from build123d import *

# Parameters (mm, degrees)
SKETCH1_W           = 584.2
SKETCH1_H           = 50.8
BOSS_EXTRUDE1_DEPTH = 9.525
SKETCH2_R           = 3.2639
CUT_EXTRUDE2_DEPTH  = 1390.972066491
SKETCH3_R           = 5.23875
CUT_EXTRUDE3_DEPTH  = 6.35
FILLET1_R           = 6.35
SKETCH4_R           = 2.4892
CUT_EXTRUDE4_DEPTH  = 1390.972066491
CHAMFER1_SIZE       = 0.79375
SHELL1_START        = 6.35
SHELL1_OUTLINE_R    = 8.8392
SHELL1_DEPTH        = 3.175


# Read off the part's stored shape, not the designer's step: Shell1
with BuildPart() as part:
    # Sketch1 → Boss-Extrude1 (new body)
    with BuildSketch(Plane.XY):
        with Locations((0, 1333.5)):
            Rectangle(SKETCH1_W, SKETCH1_H)
    extrude(amount=BOSS_EXTRUDE1_DEPTH)

    # Sketch2 → Cut-Extrude2 (cut, through all)
    with BuildSketch(Plane.XY):
        with Locations(Location((279.4, 1314.45, 0), (0, 0, 180))):
            Circle(SKETCH2_R)
        with Locations(Location((279.4, 1352.55, 0), (0, 0, 180))):
            Circle(SKETCH2_R)
    cut_extrude2 = extrude(amount=CUT_EXTRUDE2_DEPTH, mode=Mode.SUBTRACT)

    # Sketch3 → Cut-Extrude3 (cut)
    with BuildSketch(Plane(origin=(0, 0, 0), x_dir=(-1, 0, 0), z_dir=(0, 0, -1))):
        with Locations((-279.4, 1314.45)):
            Circle(SKETCH3_R)
        with Locations((-279.4, 1352.55)):
            Circle(SKETCH3_R)
    cut_extrude3 = extrude(amount=-CUT_EXTRUDE3_DEPTH, mode=Mode.SUBTRACT)

    # Fillet1
    fillet1_edges = [part.edges().sort_by_distance(p)[0] for p in [
        (292.1, 1308.1, 4.7625),
        (-292.1, 1308.1, 4.7625),
        (-292.1, 1358.9, 4.7625),
        (292.1, 1358.9, 4.7625),
    ]]
    fillet(fillet1_edges, radius=FILLET1_R)

    # Sketch4 → Cut-Extrude4 (cut, symmetric)
    with BuildSketch(Plane.XY):
        with Locations((150.8125, 1333.5)):
            Circle(SKETCH4_R)
        with Locations((188.9125, 1333.5)):
            Circle(SKETCH4_R)
    cut_extrude4 = extrude(amount=CUT_EXTRUDE4_DEPTH, both=True, mode=Mode.SUBTRACT)

    # Mirror2: Cut-Extrude2, Cut-Extrude3, Cut-Extrude4 across plane
    add(cut_extrude2.mirror(Plane(origin=(0, 0, 0), x_dir=(0, 0, 1), z_dir=(1, 0, 0))), mode=Mode.SUBTRACT)
    add(cut_extrude3.mirror(Plane(origin=(0, 0, 0), x_dir=(0, 0, 1), z_dir=(1, 0, 0))), mode=Mode.SUBTRACT)
    add(cut_extrude4.mirror(Plane(origin=(0, 0, 0), x_dir=(0, 0, 1), z_dir=(1, 0, 0))), mode=Mode.SUBTRACT)

    # Chamfer1
    chamfer1_edges = [part.edges().sort_by_distance(p)[0] for p in [
        (0, 1308.1, 0),
        (292.1, 1333.5, 0),
        (-292.1, 1333.5, 0),
        (0, 1358.9, 0),
        (290.240128061, 1357.040128061, 0),
        (290.240128061, 1309.959871939, 0),
        (-290.240128061, 1357.040128061, 0),
        (-290.240128061, 1309.959871939, 0),
    ]]
    chamfer(chamfer1_edges, length=CHAMFER1_SIZE)

    # Shell1 outline → Shell1 (cut)
    with BuildSketch(Plane.XY.offset(SHELL1_START)):
        with BuildLine():
            Line((285.75, 1324.144154247), (285.75, 1342.855845753))
            ThreePointArc((285.75, 1342.855845753), (273.89043722, 1342.354714593), (267.81125, 1352.55))
            Line((267.81125, 1352.55), (-267.81125, 1352.55))
            ThreePointArc((-267.81125, 1352.55), (-273.89043722, 1342.354714593), (-285.75, 1342.855845753))
            Line((-285.75, 1342.855845753), (-285.75, 1324.144154247))
            ThreePointArc((-285.75, 1324.144154247), (-273.89043722, 1324.645285407), (-267.81125, 1314.45))
            Line((-267.81125, 1314.45), (267.81125, 1314.45))
            ThreePointArc((267.81125, 1314.45), (273.89043722, 1324.645285407), (285.75, 1324.144154247))
        make_face()
        with Locations((-188.9125, 1333.5)):
            Circle(SHELL1_OUTLINE_R, mode=Mode.SUBTRACT)
        with Locations((-150.8125, 1333.5)):
            Circle(SHELL1_OUTLINE_R, mode=Mode.SUBTRACT)
        with Locations((150.8125, 1333.5)):
            Circle(SHELL1_OUTLINE_R, mode=Mode.SUBTRACT)
        with Locations((188.9125, 1333.5)):
            Circle(SHELL1_OUTLINE_R, mode=Mode.SUBTRACT)
    extrude(amount=SHELL1_DEPTH, mode=Mode.SUBTRACT)


solid = part.part
Check sheet for the modelled part. Datum: model origin and axes. Units: mm. A direction names the side the tool comes from. Round coordinates to 2 decimals unless told otherwise and drop trailing zeros. Order: outer loops, then holes, each group sorted by start corner. A loop starts at its lowest first (then second) coordinate and runs counter-clockwise, first axis right, second up.
Q1. Depth check by flat-ended pin: P1, Ø5, axis at x = -59.5, y = 1334.5, coming from the +Z side; P2, Ø4, axis at x = -279.4, y = 1352.55, coming from the -Z side; P3, Ø5, axis at x = 277.5, y = 1316, coming from the -Z side. Enter the tip coordinate at first touch or a pass-through.
Filled sheet:
P1: stops at z = 6.35
P2: passes through
P3: stops at z = 6.35
Q2. Set-up check for faces 1 (the face through (-277, 1355, 6.35)), 2 (the face through (-153, 1332, 9.525)), 3 (the face through (144.298, 1339.474, 7.915)): record each of +Z, -Z, +X, -X, +Y, -Y from which the full face is reachable in a straight line by a thin tool's end or side.
Filled sheet:
face 1: -Z
face 2: +Z, +X, -X, +Y, -Y
face 3: +Z
Q3. Draft check along Y on faces 4 (the face through (277, 1355, 6.35)), 5 (the face through (-1, 1313, 9.525)). Enter one of: pulls with the +Y half, pulls with the -Y half, needs draft (parallel to the pull), parting line crosses it, or undercut.
Filled sheet:
face 4: undercut
face 5: needs draft
Q4. Cross-section at B-B, the plane z = 3.75. Give the number of separate pieces and of enclosed holes in the cut face, plus the area to 3 significant figures.
Filled sheet:
separate pieces: 1
enclosed holes: 8
area: 29,200 mm2
Q5. Cross-section at A-A, the plane x = 67. Enter the section's corners in (y, z) (3 decimals), plus the area to 3 significant figures.
Filled sheet:
outline: (1308.1, 0.794) - (1308.894, 0) - (1358.106, 0) - (1358.9, 0.794) - (1358.9, 9.525) - (1352.55, 9.525) - (1352.55, 6.35) - (1314.45, 6.35) - (1314.45, 9.525) - (1308.1, 9.525) - close
area: 362 mm2
Q6. Scan lines: L1, parallel to X at y = 1314.45, z = 3.25; L2, parallel to Y at x = 279.4, z = 4.25; L3, parallel to Y at x = -86, z = 9.25. Record each from-to range of solid material in increasing order.
Filled sheet:
L1: x = -292.1 to -284.64, -274.16 to 274.16, 284.64 to 292.1
L2: y = 1308.1 to 1309.21, 1319.69 to 1347.31, 1357.79 to 1358.9
L3: y = 1308.1 to 1314.45, 1352.55 to 1358.9
